Could you check a few things on this model? Use its own coordinates, in mm. A direction names the side the tool comes from. Give positions to 0.01 mm unless a question says otherwise; leave off trailing zeros. Loops run counter-clockwise (first coordinate to the right, second up) from the corner with the lowest first, then second, coordinate; pieces in that order, holes last. Notation, with made-up numbers: M 70.5,-11 L 101.5,-11 A21 cw 101.5,13 Z; hole C 83.25,39.5 d3. An arc over 180 degrees is marked long. Return JSON: item names as keys, results as strings. Group by question number.
1. If we section it at D-D (z = 5.75): Write out the boundary of the cut face in (x, y).
2. If we section it at A-A (z = 3.5): Write out the boundary of the cut face in (x, y), plus the area to 3 significant figures.
3. For pin 1 (1.5 mm diameter, centred on y = 5.5, z = 7.5, fed in from +X); pin 2 (0.5 mm diameter, centred on x = 0, z = 2.5, fed in from -Y); pin 3 (4.5 mm diameter, centred on x = 3.5, y = 21.5, fed in from +Z), each with a flat end and sliding along its axis, tell me the tip position at first contact or that it passes through.
4. Please list where these lines run through material, in increasing order: line 1 (X direction, y = 33.5, z = 3.45); line 2 (Z direction, x = 1.1, y = 7.5); line 3 (X direction, y = 8, z = 3.75).
5. If we section it at B-B (y = 2.5): Write out the boundary of the cut face in (x, z).
6. If we section it at C-C (x = 0): Write out the boundary of the cut face in (y, z).
7. For faces 1 (the flat face through (0.5, 5, 5)), 2 (the flat face through (-3.73, 25.76, 1.48)), 3 (the flat face through (2, 10, 7)), 4 (the flat face through (-4, 0, 2)), which set-ups out of +Z, -Z, +X, -X, +Y, -Y let a thin tool reach every point of the face, with its end or its side?
8. If we mould it in two halves opening along Z, with no side actions, what happens to faces 5 (the flat face through (-5, 30, 0)), 6 (the flat face through (0, 30, 4)), 7 (the flat face through (3.5, 5, 7)), 8 (the cylindrical face through (1.98, 2.88, 5.29))? For each: +Z half, -Z half, draft (parallel to the pull), parting line (faces both ways), or undercut.
```python
from build123d import *

# Parameters (mm, degrees)
EXTRUDE_1_DEPTH     = 4
CUT_EXTRUDE_1_DEPTH = 3
SKETCH_5_R          = 1.25
CUT_EXTRUDE_2_DEPTH = 12.4
SKETCH_6_W          = 1
SKETCH_6_H          = 10
CUT_EXTRUDE_3_DEPTH = 16.3
SKETCH_9_W          = 5
SKETCH_9_H          = 10
EXTRUDE_4_DEPTH     = 3
SKETCH_10_R         = 1.25
CUT_EXTRUDE_4_DEPTH = 5.1


with BuildPart() as part:
    # 草圖1 → 填料-伸長1 (new body)
    with BuildSketch(Plane.XY):
        with BuildLine():
            Line((7.5, 0), (7.5, 52))
            ThreePointArc((7.5, 52), (0, 59.5), (-7.5, 52))
            Line((-7.5, 52), (-7.5, 0))
            Line((-7.5, 0), (7.5, 0))
        make_face()
    extrude(amount=EXTRUDE_1_DEPTH)

    # 草圖3 → 除料-伸長1 (cut)
    with BuildSketch(Plane.XY):
        with BuildLine():
            ThreePointArc((-2.5, 48.75876512), (0, 51.25876512), (2.5, 48.75876512))
            Line((2.5, 48.75876512), (5, 33.5))
            Line((5, 33.5), (2.467939071, 17.842139978))
            ThreePointArc((2.467939071, 17.842139978), (-0.200190311, 15.749263002), (-2.5, 18.24123488))
            Line((-2.5, 18.24123488), (-5, 33.5))
            Line((-5, 33.5), (-2.5, 48.75876512))
        make_face()
    extrude(amount=CUT_EXTRUDE_1_DEPTH, mode=Mode.SUBTRACT)

    # 草圖5 → 除料-伸長2 (cut)
    with BuildSketch(Plane.XY):
        with Locations((0, 33.5)):
            Circle(SKETCH_5_R)
    extrude(amount=CUT_EXTRUDE_2_DEPTH, mode=Mode.SUBTRACT)

    # 草圖6 → 除料-伸長3 (cut)
    with BuildSketch(Plane.XY):
        with Locations((0, 5)):
            Rectangle(SKETCH_6_W, SKETCH_6_H)
    extrude(amount=CUT_EXTRUDE_3_DEPTH, mode=Mode.SUBTRACT)

    # 草圖9 → 填料-伸長4 (add)
    with BuildSketch(Plane(origin=(0.5, 0, 0), x_dir=(0, 0, -1), z_dir=(1, 0, 0))):
        with Locations((-6.46178466, 5)):
            Rectangle(SKETCH_9_W, SKETCH_9_H)
    extrude(amount=EXTRUDE_4_DEPTH)

    # 草圖10 → 除料-伸長4 (cut)
    with BuildSketch(Plane(origin=(0.5, 0, 0), x_dir=(0, 0, -1), z_dir=(1, 0, 0))):
        with Locations((-6.48089233, 7.5)):
            Circle(SKETCH_10_R)
        with Locations((-6.48089233, 2.5)):
            Circle(SKETCH_10_R)
    extrude(amount=CUT_EXTRUDE_4_DEPTH, mode=Mode.SUBTRACT)


solid = part.part
```
Answer:
{
 "1": {"outline": "M 0.5,0 L 3.5,0 L 3.5,1.49 L 0.5,1.49 Z; M 0.5,3.51 L 3.5,3.51 L 3.5,6.49 L 0.5,6.49 Z; M 0.5,8.51 L 3.5,8.51 L 3.5,10 L 0.5,10 Z"},
 "2": {"outline": "M -7.5,0 L -0.5,0 L -0.5,10 L 0.5,10 L 0.5,0 L 7.5,0 L 7.5,52 A7.5 ccw -7.5,52 Z; hole C 0,33.5 d2.5", "area": "853 mm²"},
 "3": {"pin 1": "stops at x = 3.5", "pin 2": "stops at y = 10", "pin 3": "stops at z = 4"},
 "4": {"line 1": "x = -7.5 to -1.25, 1.25 to 7.5", "line 2": "z = 0 to 5.23, 7.73 to 8.96", "line 3": "x = -7.5 to -0.5, 0.5 to 7.5"},
 "5": {"outline": "M -7.5,0 L -0.5,0 L -0.5,4 L -7.5,4 Z; M 0.5,0 L 7.5,0 L 7.5,4 L 3.5,4 L 3.5,5.23 L 0.5,5.23 Z; M 0.5,7.73 L 3.5,7.73 L 3.5,8.96 L 0.5,8.96 Z"},
 "6": {"outline": "M 10,0 L 15.74,0 L 15.74,3 L 32.25,3 L 32.25,4 L 10,4 Z; M 34.75,3 L 51.26,3 L 51.26,0 L 59.5,0 L 59.5,4 L 34.75,4 Z"},
 "7": {"face 1": "+Z, -Z, -Y", "face 2": "-Z", "face 3": "+Z, +X, -X, +Y", "face 4": "+Z, -Z, +X, -X, -Y"},
 "8": {"face 5": "-Z half", "face 6": "+Z half", "face 7": "draft", "face 8": "undercut"}
}
